Geometry check sheet. Reference: drawing and pictorial views, mm from the part's lowest x, y, z. Coordinates: 2 decimals unless noted, no trailing zeros. Order: outer loops, then holes, each group sorted by start corner. A loop starts at its lowest first (then second) coordinate and runs counter-clockwise, first axis right, second up. Notation, with made-up numbers: (66, 33) -> (117, 33) arc R22 cw to (117, 67) -> close; hole circle Ø6 at (-8, -40). An arc over 180 degrees is marked (long way). Use CSV: the item, a comma, the result in double quotes. Start each with the question number.
1) Go/stop test with flat-tipped pins: pin 1 (3 mm diameter, centred on y = 11, z = 65.5, fed in from -X); pin 2 (1 mm diameter, centred on x = 88.5, y = 21, fed in from +Z); pin 3 (1.5 mm diameter, centred on x = 90, y = 16.5, fed in from +Z). Record where each tip stops, or that it passes through.
2) Sectioned sample at C-C on y = 27. Record the boundary of the cut face in (x, z).
3) Sectioned sample at A-A on z = 53.5. Record the boundary of the cut face in (x, y).
4) Release check for a two-part mould opening along X. For the marked faces 1, 2 and 3 record: released by +X, released by -X, zero draft, split by the parting line, or undercut.
5) Sectioned sample at D-D on z = 9.5. Record the boundary of the cut face in (x, y), then the cut area to 3 significant figures.
6) Scan lines: line 1 along Z through (x, y) = (53.5, 29); line 2 along Z through (x, y) = (52.5, 18.75); line 3 along Y through (x, z) = (33, 101). Record each from-to range of solid material in increasing order.
7) Sectioned sample at B-B on x = 56.5. Record the boundary of the cut face in (y, z).
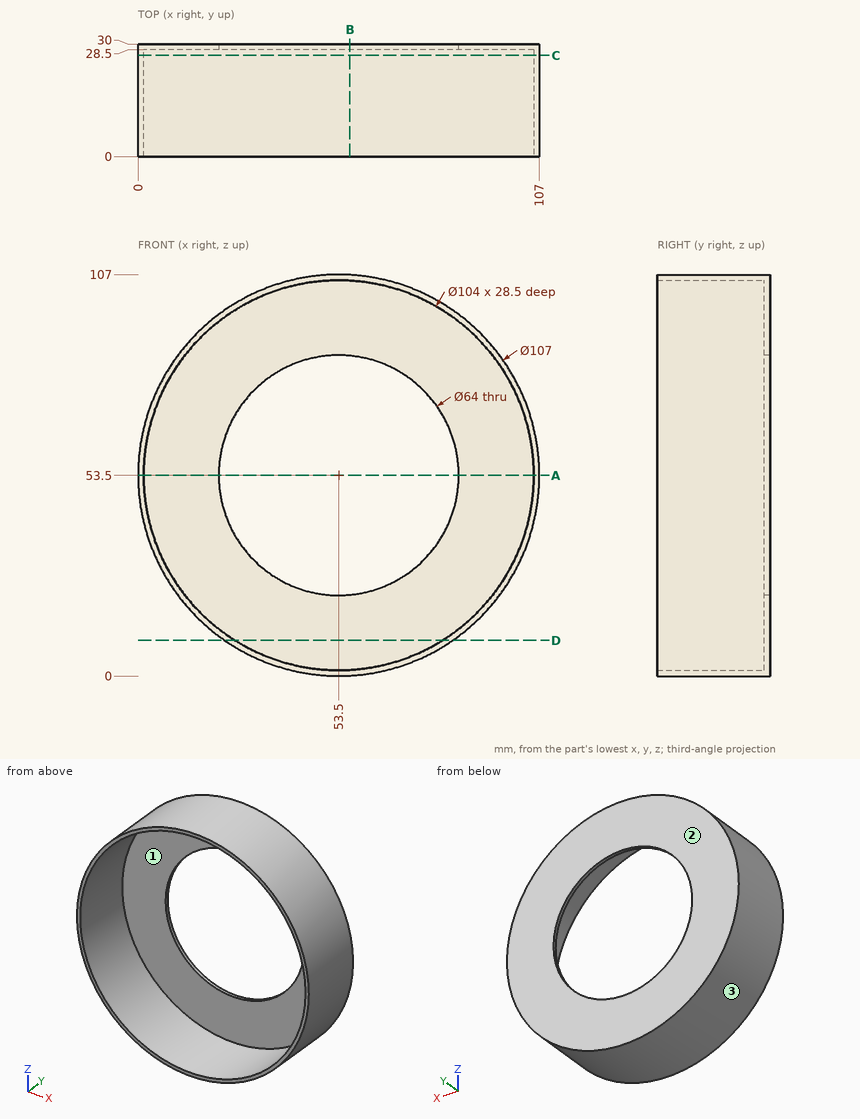
Answers follow:
1,pin 1,"stops at x = 1.04"
1,pin 2,"stops at z = 94.39"
1,pin 3,"stops at z = 93.3"
2,outline,"circle Ø107 at (53.5, 53.5); hole circle Ø104 at (53.5, 53.5)"
3,outline,"(0, 0) -> (1.5, 0) -> (1.5, 28.5) -> (21.5, 28.5) -> (21.5, 30) -> (0, 30) -> close; (85.5, 28.5) -> (105.5, 28.5) -> (105.5, 0) -> (107, 0) -> (107, 30) -> (85.5, 30) -> close"
4,face 1,"undercut"
4,face 2,"zero draft"
4,face 3,"split by the parting line"
5,outline,"(23.07, 0) -> (25.79, 0) -> (25.79, 28.5) -> (81.21, 28.5) -> (81.21, 0) -> (83.93, 0) -> (83.93, 30) -> (23.07, 30) -> close"
5,area,"246 mm²"
6,line 1,"z = 0 to 21.5, 85.5 to 107"
6,line 2,"z = 0.01 to 1.51, 105.49 to 106.99"
6,line 3,"y = 28.5 to 30"
7,outline,"(0, 0.08) -> (30, 0.08) -> (30, 21.64) -> (28.5, 21.64) -> (28.5, 1.59) -> (0, 1.59) -> close; (0, 105.41) -> (28.5, 105.41) -> (28.5, 85.36) -> (30, 85.36) -> (30, 106.92) -> (0, 106.92) -> close"
